from build123d import *

# Parameters (mm, degrees)
ESQUISSE1_W             = 44
ESQUISSE1_H             = 110
BOSS_EXTRU_1_DEPTH      = 6
ESQUISSE2_W             = 21
ESQUISSE2_H             = 6.5
ESQUISSE2_W_2           = 4
ESQUISSE2_H_2           = 75
ENL_V_MAT_EXTRU_1_DEPTH = 6
ESQUISSE4_W             = 6
ESQUISSE4_H             = 10
ESQUISSE4_H_2           = 45
ESQUISSE4_H_3           = 35
BOSS_EXTRU_2_DEPTH      = 6
ESQUISSE6_R             = 1.5
ENL_V_MAT_EXTRU_3_DEPTH = 6
ESQUISSE8_R             = 2.995
ENL_V_MAT_EXTRU_4_DEPTH = 3


with BuildPart() as part:
    # Esquisse1 → Boss.-Extru.1 (new body)
    with BuildSketch(Plane.XY):
        with Locations((22, 55)):
            Rectangle(ESQUISSE1_W, ESQUISSE1_H)
    extrude(amount=BOSS_EXTRU_1_DEPTH)

    # Esquisse2 → Enlèv. mat.-Extru.1 (cut)
    with BuildSketch(Plane.XY.offset(6)):
        with Locations((22, 10.25)):
            Rectangle(ESQUISSE2_W, ESQUISSE2_H)
        with Locations((22, 62.5)):
            Rectangle(ESQUISSE2_W_2, ESQUISSE2_H_2)
        with Locations((33.5, 62.5)):
            Rectangle(ESQUISSE2_W_2, ESQUISSE2_H_2)
        with Locations((10.5, 62.5)):
            Rectangle(ESQUISSE2_W_2, ESQUISSE2_H_2)
    extrude(amount=-ENL_V_MAT_EXTRU_1_DEPTH, mode=Mode.SUBTRACT)

    # Esquisse4 → Boss.-Extru.2 (add)
    with BuildSketch(Plane.XY.offset(6)):
        with Locations((-3, 105)):
            Rectangle(ESQUISSE4_W, ESQUISSE4_H)
        with Locations((-3, 67.5)):
            Rectangle(ESQUISSE4_W, ESQUISSE4_H_2)
        with Locations((-3, 17.5)):
            Rectangle(ESQUISSE4_W, ESQUISSE4_H_3)
        with Locations((47, 17.5)):
            Rectangle(ESQUISSE4_W, ESQUISSE4_H_3)
        with Locations((47, 67.5)):
            Rectangle(ESQUISSE4_W, ESQUISSE4_H_2)
        with Locations((47, 105)):
            Rectangle(ESQUISSE4_W, ESQUISSE4_H)
    extrude(amount=-BOSS_EXTRU_2_DEPTH)

    # Esquisse6 → Enlèv. mat.-Extru.3 (cut)
    with BuildSketch(Plane.XY.offset(6)):
        with Locations((21, 3)):
            Circle(ESQUISSE6_R)
    extrude(amount=-ENL_V_MAT_EXTRU_3_DEPTH, mode=Mode.SUBTRACT)

    # Esquisse8 → Enlèv. mat.-Extru.4 (cut)
    with BuildSketch(Plane.XY.offset(6)):
        with Locations((21, 3)):
            Circle(ESQUISSE8_R)
    extrude(amount=-ENL_V_MAT_EXTRU_4_DEPTH, mode=Mode.SUBTRACT)


solid = part.part
Input: part model. Units: mm. Frame: model coordinates. A direction names the side the tool comes from. Round coordinates to 2 decimals unless told otherwise and drop trailing zeros. Loops run counter-clockwise (first coordinate to the right, second up) from the corner with the lowest first, then second, coordinate; pieces in that order, holes last. Notation, with made-up numbers: M 12.25,56.25 L 44.25,56.25 A14 ccw 44.25,65.25 Z; hole C 43.5,72 d4. An arc over 180 degrees is marked long. Answer as CSV lines item,"result". Start each with the question number.
(1) Section C-C, the plane y = 95. Output: boundary loops of the cut face in (x, z), plus the area to 3 significant figures.
(2) Draft query along Y for faces 1 (the flat face through (-6, 67, 3)), 2 (the flat face through (22, 110, 3)), 3 (the flat face through (22.3, 1.7, 3)). Return one class per face: released by +Y, released by -Y, zero draft, split by the parting line, or undercut.
(3) First-contact query: pin 1 (2.5 mm diameter, centred on x = 21, y = 3, fed in from +Z). Flat tip, straight axial feed; report the tip coordinate or a pass-through.
(4) Section D-D, the plane y = 54.5. Output: boundary loops of the cut face in (x, z), plus the area to 3 significant figures.
(5) Section A-A, the plane y = 3. Output: boundary loops of the cut face in (x, z) (3 decimals), plus the area to 3 significant figures.
(6) Line query: line 1 (X direction, y = 59, z = 1.15); line 2 (X direction, y = 99, z = 2.25); line 3 (Y direction, x = 26, z = 3.95). Output: solid intervals per line, ascending. Write a range as [from, to].
(7) Section B-B, the plane x = 21. Output: boundary loops of the cut face in (y, z) (3 decimals), plus the area to 3 significant figures.
(8) Reachability of faces 4 (the flat face through (47, 35, 3)), 5 (the flat face through (-3, 100, 3)), 6 (the flat face through (33, 25, 3)) from +Z, -Z, +X, -X, +Y, -Y: full face, straight path, thin tool, end or side. Return the list, or none.
Values found:
1,outline,"M 0,0 L 8.5,0 L 8.5,6 L 0,6 Z; M 12.5,0 L 20,0 L 20,6 L 12.5,6 Z; M 24,0 L 31.5,0 L 31.5,6 L 24,6 Z; M 35.5,0 L 44,0 L 44,6 L 35.5,6 Z"
1,area,"192 mm²"
2,face 1,"zero draft"
2,face 2,"released by +Y"
2,face 3,"undercut"
3,pin 1,"passes through"
4,outline,"M -6,0 L 8.5,0 L 8.5,6 L -6,6 Z; M 12.5,0 L 20,0 L 20,6 L 12.5,6 Z; M 24,0 L 31.5,0 L 31.5,6 L 24,6 Z; M 35.5,0 L 50,0 L 50,6 L 35.5,6 Z"
4,area,"264 mm²"
5,outline,"M -6,0 L 19.5,0 L 19.5,3 L 18.005,3 L 18.005,6 L -6,6 Z; M 22.5,0 L 50,0 L 50,6 L 23.995,6 L 23.995,3 L 22.5,3 Z"
5,area,"309 mm²"
6,line 1,"x = [-6, 8.5], [12.5, 20], [24, 31.5], [35.5, 50]"
6,line 2,"x = [0, 8.5], [12.5, 20], [24, 31.5], [35.5, 44]"
6,line 3,"y = [0, 7], [13.5, 110]"
7,outline,"M 0,0 L 1.5,0 L 1.5,3 L 0.005,3 L 0.005,6 L 0,6 Z; M 4.5,0 L 7,0 L 7,6 L 5.995,6 L 5.995,3 L 4.5,3 Z; M 13.5,0 L 25,0 L 25,6 L 13.5,6 Z; M 100,0 L 110,0 L 110,6 L 100,6 Z"
7,area,"144 mm²"
8,face 4,"+Z, -Z, +X"
8,face 5,"+Z, -Z, -X"
8,face 6,"+Z, -Z"
